Read the model definition and answer for the solid it produces. Units are mm, in the model's axes. A direction names the side the tool comes from. Round coordinates to 2 decimals unless told otherwise and drop trailing zeros. Order: outer loops, then holes, each group sorted by start corner. A loop starts at its lowest first (then second) coordinate and runs counter-clockwise, first axis right, second up. Notation, with made-up numbers: (63, 49) - (69, 49) arc R24 cw to (69, 67) - close; hole circle Ø10 at (21.25, 85). An arc over 180 degrees is marked (long way). Put each result on its own line as item: value. Start each with the question number.
Q1. Section A-A on z = 9.5 is taken. Give the vertices of the cut face in (x, y), then the cut area to 3 significant figures.
Q2. Section C-C on x = 16 is taken. Give the vertices of the cut face in (y, z).
Q3. Each of these flat-tipped pins is pushed along its axis until it touches: pin 1 Ø4 at (x, z) = (23, 33.5) entering from -Y; pin 2 Ø8 at (x, y) = (-10, 10.5) entering from -Z; pin 3 Ø12 at (y, z) = (-20, 57.5) entering from -X; pin 4 Ø6 at (y, z) = (-8.5, 21) entering from -X. Where does it stop, or does it pass through?
Q4. Section D-D on x = -12 is taken. State how many separate pieces and enclosed holes the cut face has, then the cut area to 3 significant figures.
Q5. For a pull along X with two mould halves and no side action, classify faces 1 (the face through (-11.13, 25.54, 85.61)), 2 (the face through (16.4, -6.9, 0)), 3 (the face through (-28.69, -16.26, 49.3)) as pulls with the +X half, pulls with the -X half, needs draft (parallel to the pull), parting line crosses it, or undercut.
Q6. Section B-B on y = -13 is taken. Give the vertices of the cut face in (x, z), then the cut area to 3 significant figures.
Q7. Find the intervals of material crossed by line 1 along Y through (x, z) = (0, 66); line 2 along Z through (x, y) = (13, 20); line 3 along X through (y, z) = (-28.5, 87.5), in increasing order. Write a range as from..to.
Q8. Which of the six approach directions +Z, -Z, +X, -X, +Y, -Y give full straight-line access (tool end or side, diameter ignored) to faces 4 (the face through (-11.106, 25.541, 13.028)), 5 (the face through (-18.45, 3.2, 50.7))?
from build123d import *

# Parameters (mm, degrees)
EXTRUDE_1_DEPTH     = 100
SKETCH_2_R          = 18.469515879
CUT_EXTRUDE_1_DEPTH = 100
CUT_EXTRUDE_6_DEPTH = 126.697486666


with BuildPart() as part:
    # 草图1 → 凸台-拉伸1 (new body)
    with BuildSketch(Plane.XY):
        Polygon((38.078399894, 0), (19.039199947, 32.976861644), (-19.039199947, 32.976861644), (-38.078399894, 0), (-19.039199947, -32.976861644), (19.039199947, -32.976861644), align=None)
    extrude(amount=EXTRUDE_1_DEPTH)

    # 草图2 → 切除-拉伸1 (cut)
    with BuildSketch(Plane.XY.offset(100)):
        with Locations((0, 2.389391374)):
            Circle(SKETCH_2_R)
    extrude(amount=-CUT_EXTRUDE_1_DEPTH, mode=Mode.SUBTRACT)

    # 草图7 → 切除-拉伸6 (cut, through all)
    with BuildSketch(Plane(origin=(0, 32.976861644, 0), x_dir=(1, 0, 0), z_dir=(0, 1, 0))):
        Polygon((6.96455573, -36.71488632), (-7.562692597, -36.803663943), (-14.749433085, -49.429018853), (-7.408925244, -61.965596141), (7.118323083, -61.876818518), (14.305063571, -49.251463608), align=None)
        Polygon((6.96455573, -6.71488632), (-7.562692597, -6.803663943), (-14.749433085, -19.429018853), (-7.408925244, -31.965596141), (7.118323083, -31.876818518), (14.305063571, -19.251463608), align=None)
        Polygon((6.96455573, -66.71488632), (-7.562692597, -66.803663943), (-14.749433085, -79.429018853), (-7.408925244, -91.965596141), (7.118323083, -91.876818518), (14.305063571, -79.251463608), align=None)
    extrude(amount=-CUT_EXTRUDE_6_DEPTH, mode=Mode.SUBTRACT)


solid = part.part
Findings:
1. outline: (-38.08, 0) - (-19.04, -32.98) - (-9.1, -32.98) - (-9.1, -13.68) arc R18.47 cw to (-9.1, 18.46) - (-9.1, 32.98) - (-19.04, 32.98) - close; (8.6, -32.98) - (19.04, -32.98) - (38.08, 0) - (19.04, 32.98) - (8.6, 32.98) - (8.6, 18.74) arc R18.47 cw to (8.6, -13.96) - close
1. area: 2,160 mm2
2. outline: (-32.98, 0) - (-6.84, 0) - (-6.84, 100) - (-32.98, 100) - close; (11.62, 0) - (32.98, 0) - (32.98, 100) - (11.62, 100) - close
3. pin 1: y = -29.58
3. pin 2: through
3. pin 3: x = -30
3. pin 4: x = -34.9
4. separate pieces: 8
4. enclosed holes: 0
4. area: 2,710 mm2
5. face 1: undercut
5. face 2: needs draft
5. face 3: pulls with the -X half
6. outline: (-30.57, 0) - (-10.21, 0) - (-10.21, 11.46) - (-14.75, 19.43) - (-10.21, 27.18) - (-10.21, 41.46) - (-14.75, 49.43) - (-10.21, 57.18) - (-10.21, 71.46) - (-14.75, 79.43) - (-10.21, 87.18) - (-10.21, 100) - (-30.57, 100) - close; (10.21, 0) - (30.57, 0) - (30.57, 100) - (10.21, 100) - (10.21, 86.44) - (14.31, 79.25) - (10.21, 72.26) - (10.21, 56.44) - (14.31, 49.25) - (10.21, 42.26) - (10.21, 26.44) - (14.31, 19.25) - (10.21, 12.26) - close
6. area: 3,880 mm2
7. line 1: -32.98..-16.08, 20.86..32.98
7. line 2: 0..17.02, 21.54..47.02, 51.54..77.02, 81.54..100
7. line 3: -21.62..-10.02, 9.61..21.62
8. face 4: +Y, -Y
8. face 5: +Z, -Z
